Model file for the job. Use its own axes, mm. A direction names the side the tool comes from. Round coordinates to 2 decimals unless told otherwise and drop trailing zeros. Write each loop counter-clockwise with the first axis right and the second up, starting at its lowest first coordinate (ties: lowest second). Pieces come first, ordered by that corner, then holes. Notation, with made-up numbers: (0, -39) - (19, -39) arc R25 cw to (19, -13) - close; hole circle Ø3 at (29, 29.25). An arc over 180 degrees is marked (long way). One line per item, written item: value.
from build123d import *

# Parameters (mm, degrees)
BOSS_EXTRUDE1_DEPTH = 1.984375
CHAMFER2_SIZE       = 1.984375
CHAMFER4_SIZE       = 1.984375
CHAMFER5_SIZE       = 1.984375
FILLET1_R           = 0.25


with BuildPart() as part:
    # Sketch1 → Boss-Extrude1 (new body)
    with BuildSketch(Plane.XY):
        Polygon((0, 0), (-20, 0), (-10, 17.320508076), align=None)
        Polygon((-14.803847577, 3), (-10, 11.320508076), (-5.196152423, 3), align=None, mode=Mode.SUBTRACT)
    extrude(amount=BOSS_EXTRUDE1_DEPTH)

    # Chamfer2
    chamfer2_edges = [part.edges().sort_by_distance(p)[0] for p in [
        (-20, 0, 0.9921875),
    ]]
    chamfer(chamfer2_edges, length=CHAMFER2_SIZE)

    # Chamfer4
    chamfer4_edges = [part.edges().sort_by_distance(p)[0] for p in [
        (0, 0, 0.9921875),
    ]]
    chamfer(chamfer4_edges, length=CHAMFER4_SIZE)

    # Chamfer5
    chamfer5_edges = [part.edges().sort_by_distance(p)[0] for p in [
        (-10, 17.320508076, 0.9921875),
    ]]
    chamfer(chamfer5_edges, length=CHAMFER5_SIZE)

    # Fillet1
    fillet1_edges = [part.edges().sort_by_distance(p)[0] for p in [
        (-14.803847577, 3, 0.9921875),
        (-5.196152423, 3, 0.9921875),
        (-10, 11.320508076, 0.9921875),
    ]]
    fillet(fillet1_edges, radius=FILLET1_R)


solid = part.part
1. Wall check: probe 1 along Y at (x, z) = (-10, 0.55); probe 2 along Y at (x, z) = (-6.75, 1.6); probe 3 along X at (y, z) = (3.75, 0.95). Give the ranges that are in metal, low to high. Write a range as [from, to].
Report:
probe 1: [0, 3], [11.07, 15.6]
probe 2: [0, 3], [5.69, 11.69]
probe 3: [-17.83, -14.37], [-5.63, -2.17]
2. Tool access for faces 1 (the face through (-10, 3, 1)), 2 (the face through (-18.52, 0.87, 0.98)): list every direction of +Z, -Z, +X, -X, +Y, -Y with a clear straight run to the whole face (end or side of a thin tool).
Report:
face 1: +Z, -Z
face 2: +Z, -Z, -X, -Y
3. Band-saw the part on C-C on y = 4.25. Write the cut outline in (x, z), plus the area to 3 significant figures.
Report:
outline: (-17.55, 0) - (-14.08, 0) - (-14.08, 1.98) - (-17.55, 1.98) - close; (-5.92, 0) - (-2.45, 0) - (-2.45, 1.98) - (-5.92, 1.98) - close
area: 13.7 mm²
4. Mould opens along Y. For faces 3 (the face through (-15.06, 8.56, 0.98)), 4 (the face through (-12.43, 7.11, 0.98)), 5 (the face through (-10, 0, 1)) say: released by +Y, released by -Y, zero draft, split by the parting line, or undercut.
Report:
face 3: released by +Y
face 4: undercut
face 5: released by -Y
5. Band-saw the part on A-A on x = -7.5. Write the cut outline in (y, z).
Report:
outline: (0, 0) - (3, 0) - (3, 1.98) - (0, 1.98) - close; (6.99, 0) - (12.99, 0) - (12.99, 1.98) - (6.99, 1.98) - close
6. Band-saw the part on D-D on x = -4.75. Write the cut outline in (y, z).
Report:
outline: (0, 0) - (8.23, 0) - (8.23, 1.98) - (0, 1.98) - close
